Geometry: see drawing. Coordinates: mm, zero at the bounding-box minimum. A direction names the side the tool comes from. Round coordinates to 2 decimals unless told otherwise and drop trailing zeros. Order: outer loops, then holes, each group sorted by start corner. A loop starts at its lowest first (then second) coordinate and runs counter-clockwise, first axis right, second up. Notation, with made-up numbers: (-2, -30.5) -> (17, -30.5) arc R35 ccw to (17, 6.5) -> close; hole circle Ø9 at (41.5, 74.5). An arc over 180 degrees is marked (long way). One line per item, written item: value. Start each with the question number.
1) Section C-C (z = 6). Return the cut outline in (x, y).
2) Section D-D (z = 1.5). Return the cut outline in (x, y), and give its area (3 significant figures).
3) Section A-A (y = 1). Return the cut outline in (x, z), and give its area (3 significant figures).
4) Mould query, pull axis Z, two halves, no side actions, for the marked faces 4, 5, 6 and 7. Classes: pulls with the +Z half, pulls with the -Z half, needs draft (parallel to the pull), parting line crosses it, or undercut.
5) Ray query, L1, parallel to X at y = 2.9, z = 6; L2, parallel to X at y = 6.75, z = 7.5; L3, parallel to Z at x = 8, y = 1.8. Return the intervals inside material, ascending.
6) Pin query (flat end, axial travel): P1, Ø2, axis at y = 7, z = 10, coming from the +X side; P2, Ø5, axis at x = 8, z = 6, coming from the +Y side. Return the tip coordinate at first contact, or that it passes through.
7) Section B-B (x = 8). Return the cut outline in (y, z), and give its area (3 significant figures).
8) Reachability of the marked faces 1, 2 and 3 from +Z, -Z, +X, -X, +Y, -Y: full face, straight path, thin tool, end or side. Return the list, or none.
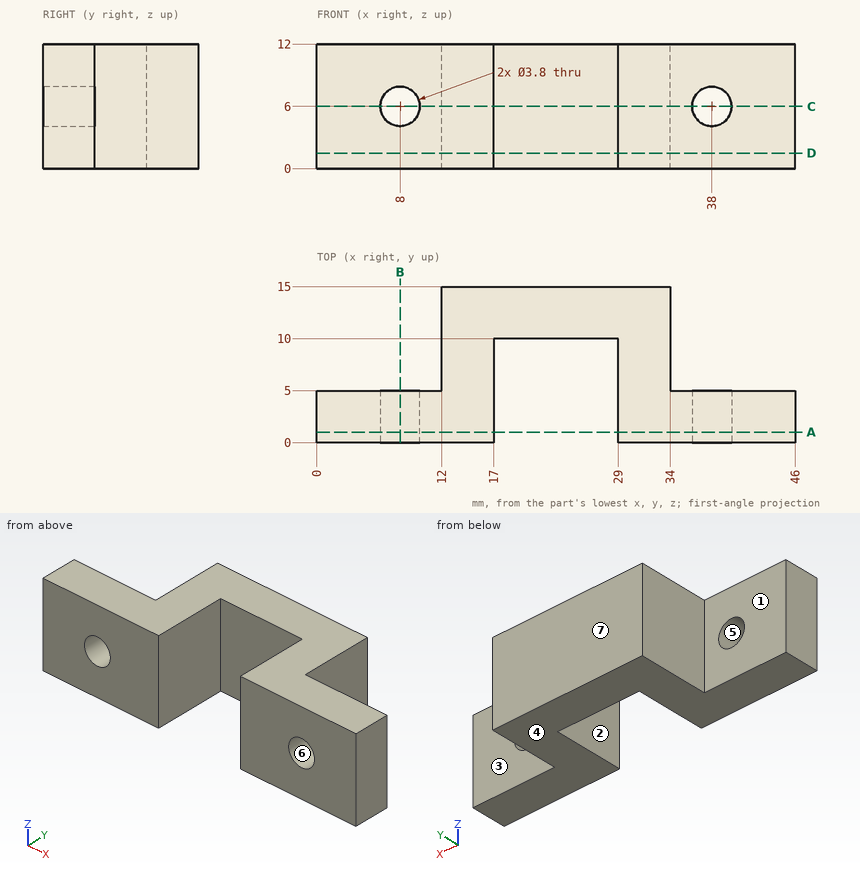
Findings:
1. outline: (0, 0) -> (6.1, 0) -> (6.1, 5) -> (0, 5) -> close; (9.9, 0) -> (17, 0) -> (17, 10) -> (29, 10) -> (29, 0) -> (36.1, 0) -> (36.1, 5) -> (34, 5) -> (34, 15) -> (12, 15) -> (12, 5) -> (9.9, 5) -> close; (39.9, 0) -> (46, 0) -> (46, 5) -> (39.9, 5) -> close
2. outline: (0, 0) -> (17, 0) -> (17, 10) -> (29, 10) -> (29, 0) -> (46, 0) -> (46, 5) -> (34, 5) -> (34, 15) -> (12, 15) -> (12, 5) -> (0, 5) -> close
2. area: 330 mm2
3. outline: (0, 0) -> (17, 0) -> (17, 12) -> (0, 12) -> close; (29, 0) -> (46, 0) -> (46, 12) -> (29, 12) -> close; hole circle Ø3.8 at (8, 6); hole circle Ø3.8 at (38, 6)
3. area: 385 mm2
4. face 4: pulls with the -Z half
4. face 5: undercut
4. face 6: undercut
4. face 7: needs draft
5. L1: 0 to 6.1, 9.9 to 17, 29 to 36.1, 39.9 to 46
5. L2: 12 to 17, 29 to 34
5. L3: 0 to 4.1, 7.9 to 12
6. P1: x = 34
6. P2: y = 5
7. outline: (0, 0) -> (5, 0) -> (5, 4.1) -> (0, 4.1) -> close; (0, 7.9) -> (5, 7.9) -> (5, 12) -> (0, 12) -> close
7. area: 41.0 mm2
8. face 1: +Z, -Z, -X, +Y
8. face 2: +Z, -Z, -Y
8. face 3: +Z, -Z, +X, +Y
